Work out the finished part from the listing and answer in its coordinate system (mm). Coordinates: 2 decimals unless noted, no trailing zeros. Write each loop counter-clockwise with the first axis right and the second up, starting at its lowest first coordinate (ties: lowest second). Pieces come first, ordered by that corner, then holes. Notation, with made-up numbers: M -12,16.5 L 30,16.5 A19 ccw 30,51.5 Z; hole C 37,13 d4. An arc over 180 degrees is marked long. Answer as CSV lines item,"result". Start each with the question number.
(1) Flat-ended cylindrical pins translate along their axes: P1, Ø1.5, axis at x = -19, y = 2, coming from the -Z side; P2, Ø1.5, axis at y = 1, z = 32, coming from the -X side. Find the tip coordinate at first contact, or state that the pin passes through.
(2) A cutting plane is placed at A-A on z = 0. Give the vertices of the cut face in (x, y) (3 decimals).
(3) A cutting plane is placed at D-D on z = -20.32. Give the vertices of the cut face in (x, y) (3 decimals), then the cut area to 3 significant figures.
(4) A cutting plane is placed at B-B on x = 0. Give the vertices of the cut face in (y, z) (3 decimals), then the cut area to 3 significant figures.
(5) The mould has two halves that part along Z. Classify faces 1 (the cylindrical face through (-33.35, 1.57, 20.24)), 2 (the cylindrical face through (42.397, 1.565, -13.352)), 3 (the flat face through (9.3, 0, 29)), 4 (the cylindrical face through (-0.85, 1.57, -39)): released by +Z, released by -Z, zero draft, split by the parting line, or undercut.
(6) A cutting plane is placed at C-C on y = 0.9. Give the vertices of the cut face in (x, z), then the cut area to 3 significant figures.
(7) Find the intervals of material crossed by L1, parallel to Z at x = 0, y = 2.45; L2, parallel to X at y = 1.55, z = -20.32; L3, parallel to X at y = 1.55, z = 0, in increasing order. Write a range as [from, to].
from build123d import *

# Parameters (mm, degrees)
SKETCH1_R                 = 44.45
SKETCH1_R_2               = 30.275917709
BOSS_EXTRUDE1_DEPTH       = 3.175
F_6_CLEARANCE_HOLE1_D     = 3.6957
F_6_CLEARANCE_HOLE1_DEPTH = 3.176
CIRPATTERN1_COUNT         = 6


with BuildPart() as part:
    # Sketch1 → Boss-Extrude1 (new body)
    with BuildSketch(Plane(origin=(0, 0, 0), x_dir=(1, 0, 0), z_dir=(0, 1, 0))):
        Circle(SKETCH1_R)
        Circle(SKETCH1_R_2, mode=Mode.SUBTRACT)
    extrude(amount=BOSS_EXTRUDE1_DEPTH)

    # #6 Clearance Hole1
    with Locations(Plane(origin=(0, 3.175, 0), x_dir=(1, 0, 0), z_dir=(0, 1, 0))):
        with Locations((0, 40.64)):
            f_6_clearance_hole1 = Hole(F_6_CLEARANCE_HOLE1_D / 2, depth=F_6_CLEARANCE_HOLE1_DEPTH)

    # CirPattern1: #6 Clearance Hole1 ×6 about axis
    cirpattern1_axis = Axis((0, 0, 0), (0, 1, 0))
    for i in range(1, CIRPATTERN1_COUNT):
        add(f_6_clearance_hole1.rotate(cirpattern1_axis, i * 360 / CIRPATTERN1_COUNT), mode=Mode.SUBTRACT)


solid = part.part
Here are the results:
1,P1,"stops at z = -40.53"
1,P2,"stops at x = -31.61"
2,outline,"M -44.45,0 L -30.276,0 L -30.276,3.175 L -44.45,3.175 Z; M 30.276,0 L 44.45,0 L 44.45,3.175 L 30.276,3.175 Z"
3,outline,"M -39.534,0 L -37.043,0 L -37.043,3.175 L -39.534,3.175 Z; M -33.347,0 L -22.444,0 L -22.444,3.175 L -33.347,3.175 Z; M 22.444,0 L 33.347,0 L 33.347,3.175 L 22.444,3.175 Z; M 37.043,0 L 39.534,0 L 39.534,3.175 L 37.043,3.175 Z"
3,area,"85.1 mm^2"
4,outline,"M 0,-44.45 L 3.175,-44.45 L 3.175,-42.488 L 0,-42.488 Z; M 0,-38.792 L 3.175,-38.792 L 3.175,-30.276 L 0,-30.276 Z; M 0,30.276 L 3.175,30.276 L 3.175,38.792 L 0,38.792 Z; M 0,42.488 L 3.175,42.488 L 3.175,44.45 L 0,44.45 Z"
4,area,"66.5 mm^2"
5,face 1,"undercut"
5,face 2,"split by the parting line"
5,face 3,"zero draft"
5,face 4,"undercut"
6,outline,"C 0,0 d88.9; hole C -35.2,-20.32 d3.7; hole C -35.2,20.32 d3.7; hole C 0,0 d60.55; hole C 0,-40.64 d3.7; hole C 0,40.64 d3.7; hole C 35.2,-20.32 d3.7; hole C 35.2,20.32 d3.7"
6,area,"3,260 mm^2"
7,L1,"z = [-44.45, -42.49], [-38.79, -30.28], [30.28, 38.79], [42.49, 44.45]"
7,L2,"x = [-39.53, -37.04], [-33.35, -22.44], [22.44, 33.35], [37.04, 39.53]"
7,L3,"x = [-44.45, -30.28], [30.28, 44.45]"
